Verification items for the finished model (mm, model axes). Give positions to 0.01 mm unless a question says otherwise; leave off trailing zeros. Order: outer loops, then holes, each group sorted by start corner. A loop starts at its lowest first (then second) coordinate and runs counter-clockwise, first axis right, second up.
from build123d import *

# Parameters (mm, degrees)
SKETCH1_R                 = 70
BOSS_EXTRUDE1_DEPTH       = 10
BOSS_EXTRUDE2_START       = -3
BOSS_EXTRUDE2_OUTLINE_R   = 65
BOSS_EXTRUDE2_DEPTH       = 3
BOSS_EXTRUDE3_DEPTH       = 5
M4X0_7_TAPPED_HOLE1_D     = 3.3
M4X0_7_TAPPED_HOLE1_DEPTH = 10.1
M4X0_7_TAPPED_HOLE1_TIP   = 0.991420021
F_8_0MM_DOWEL_HOLE1_D     = 8
F_8_0MM_DOWEL_HOLE2_D     = 8
M4X0_7_TAPPED_HOLE2_D     = 3.3
M4X0_7_TAPPED_HOLE2_DEPTH = 10.1
M4X0_7_TAPPED_HOLE2_TIP   = 0.991420021


# Read off the part's stored shape, not the designer's step: Boss-Extrude2
with BuildPart() as part:
    # Sketch1 → Boss-Extrude1 (new body)
    with BuildSketch(Plane(origin=(0, 0, 0), x_dir=(1, 0, 0), z_dir=(0, 1, 0))):
        with Locations(Location((0, 0, 0), (0, 0, 270))):
            Circle(SKETCH1_R)
    extrude(amount=BOSS_EXTRUDE1_DEPTH)

    # Boss-Extrude2 outline → Boss-Extrude2 (add)
    with BuildSketch(Plane(origin=(0, 0, 0), x_dir=(1, 0, 0), z_dir=(0, 1, 0)).offset(BOSS_EXTRUDE2_START)):
        Circle(BOSS_EXTRUDE2_OUTLINE_R)
    extrude(amount=BOSS_EXTRUDE2_DEPTH)

    # Sketch3 → Boss-Extrude3 (add, symmetric)
    with BuildSketch(Plane.XY):
        with BuildLine():
            Line((-25, 55), (-25, 5))
            Line((-25, 5), (-90, 5))
            Line((-90, 5), (-102.792798963, 41.896399481))
            ThreePointArc((-102.792798963, 41.896399481), (-71.644096684, 94.444340269), (-25, 55))
        make_face()
    extrude(amount=BOSS_EXTRUDE3_DEPTH, both=True)

    # M4x0.7 Tapped Hole1
    with Locations(Plane(origin=(0, 10, 0), x_dir=(1, 0, 0), z_dir=(0, 1, 0))):
        with Locations((5, 23.62), (52.24, 23.62), (52.24, -23.62), (5, -23.62)):
            Hole(M4X0_7_TAPPED_HOLE1_D / 2, depth=M4X0_7_TAPPED_HOLE1_DEPTH)
            with Locations((0, 0, -(M4X0_7_TAPPED_HOLE1_DEPTH + M4X0_7_TAPPED_HOLE1_TIP / 2))):  # 118° drill point
                Cone(0, M4X0_7_TAPPED_HOLE1_D / 2, M4X0_7_TAPPED_HOLE1_TIP, mode=Mode.SUBTRACT)

    # Ø8.0mm Dowel Hole1 (through all)
    with Locations(Plane(origin=(0, 10, 0), x_dir=(1, 0, 0), z_dir=(0, 1, 0))):
        with Locations((28.62, 0)):
            Hole(F_8_0MM_DOWEL_HOLE1_D / 2)

    # Ø8.0mm Dowel Hole2 (through all)
    with Locations(Plane.XY.offset(5)):
        with Locations((-65, 57.639293091)):
            Hole(F_8_0MM_DOWEL_HOLE2_D / 2)

    # M4x0.7 Tapped Hole2
    with Locations(Plane(origin=(-106.523745818, 66.238796536, 5), x_dir=(1, 0, 0), z_dir=(0, 0, 1))):
        with Locations((17.903745818, 15.020496555), (65.143745818, 15.020496555), (65.143745818, -32.219503445), (17.903745818, -32.219503445)):
            Hole(M4X0_7_TAPPED_HOLE2_D / 2, depth=M4X0_7_TAPPED_HOLE2_DEPTH)
            with Locations((0, 0, -(M4X0_7_TAPPED_HOLE2_DEPTH + M4X0_7_TAPPED_HOLE2_TIP / 2))):  # 118° drill point
                Cone(0, M4X0_7_TAPPED_HOLE2_D / 2, M4X0_7_TAPPED_HOLE2_TIP, mode=Mode.SUBTRACT)


solid = part.part
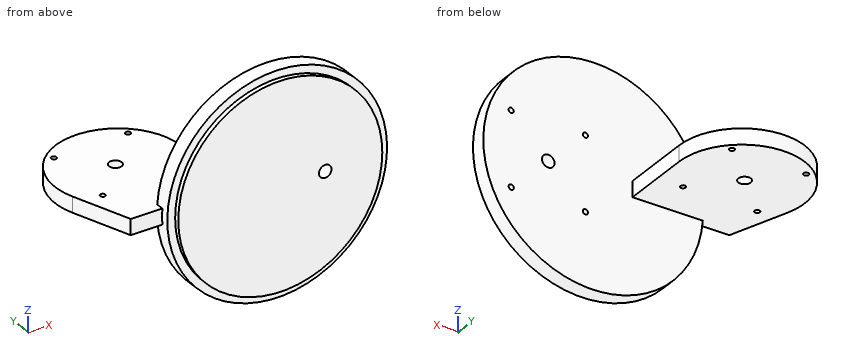
(1) Go/stop test with flat-tipped pins: pin 1 (24 mm diameter, centred on x = -57, y = 69, fed in from -Z); pin 2 (9 mm diameter, centred on x = 28.62, z = 0, fed in from +Y); pin 3 (4 mm diameter, centred on y = 43, z = -8.5, fed in from -X); pin 4 (5 mm diameter, centred on x = -76, z = 2.5, fed in from -Y). Record where each tip stops, or that it passes through.
Solved:
pin 1: stops at z = -5
pin 2: stops at y = 10
pin 3: passes through
pin 4: stops at y = 5
(2) Section check D-D, the plane z = -38. Enter the section's corners in (x, y).
Solved:
outline: (-58.79, 0) - (-52.74, 0) - (-52.74, -3) - (52.74, -3) - (52.74, 0) - (58.79, 0) - (58.79, 10) - (-58.79, 10) - close
(3) Section check B-B, the plane x = 28.62. Enter the section's corners in (y, z), then the cut area to 3 significant figures.
Solved:
outline: (-3, -58.36) - (0, -58.36) - (0, -63.88) - (10, -63.88) - (10, -4) - (-3, -4) - close; (-3, 4) - (10, 4) - (10, 63.88) - (0, 63.88) - (0, 58.36) - (-3, 58.36) - close
area: 1,520 mm2
(4) Section check A-A, the plane z = 0. Enter the section's corners in (x, y), then the cut area to 3 significant figures.
Solved:
outline: (-102.79, 41.9) - (-90, 5) - (-70, 5) - (-70, 0) - (-65, 0) - (-65, -3) - (24.62, -3) - (24.62, 10) - (-25, 10) - (-25, 55) arc R40 ccw (long way) to start; (32.62, -3) - (65, -3) - (65, 0) - (70, 0) - (70, 10) - (32.62, 10) - close; hole circle Ø3.3 at (-88.62, 34.02); hole circle Ø3.3 at (-88.62, 81.26); hole circle Ø8 at (-65, 57.64); hole circle Ø3.3 at (-41.38, 34.02); hole circle Ø3.3 at (-41.38, 81.26)
area: 7,560 mm2
(5) Section check C-C, the plane x = 0. Enter the section's corners in (y, z).
Solved:
outline: (-3, -65) - (0, -65) - (0, -70) - (10, -70) - (10, 70) - (0, 70) - (0, 65) - (-3, 65) - close
(6) Scan lines: line 1 (Z direction, x = -76, y = 45); line 2 (Y direction, x = 4, z = -26.5); line 3 (X direction, y = 2, z = 23.62). Record each from-to range of solid material in increasing order.
Solved:
line 1: z = -5 to 5
line 2: y = -3 to 10
line 3: x = -65.89 to 3.35, 6.65 to 50.59, 53.89 to 65.89
